Geometry: see drawing. Coordinates: mm, zero at the bounding-box minimum. A direction names the side the tool comes from. Give positions to 0.01 mm unless a question says otherwise; leave off trailing zeros. Order: outer loops, then holes, each group sorted by start corner. A loop starts at its lowest first (then second) coordinate and runs counter-clockwise, first axis right, second up. Notation, with made-up numbers: (88.5, 46) - (120.5, 46) arc R20 cw to (120.5, 66) - close; hole circle Ø2 at (23, 38.5). An arc over 180 degrees is marked (long way). One line per item, written item: value.
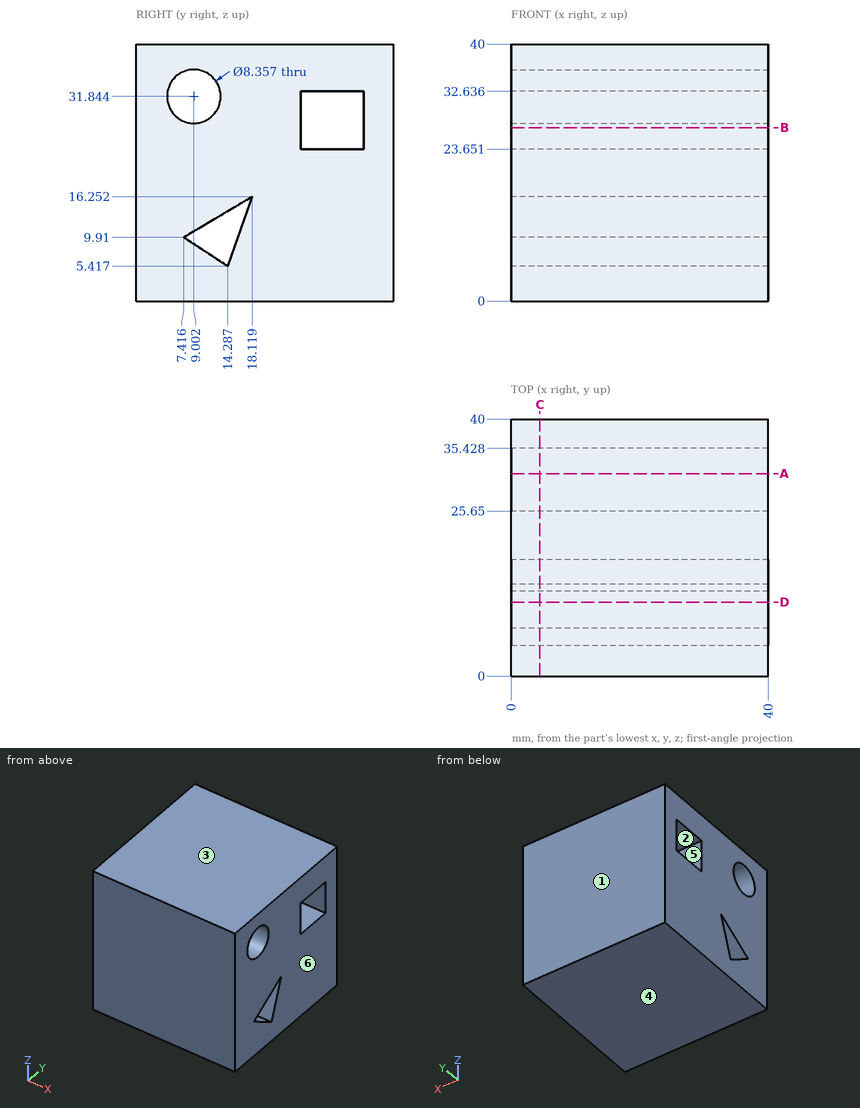
1) Section C-C, the plane x = 4.5. Return loops of the section in (y, z).
Answers below:
outline: (0, 0) - (40, 0) - (40, 40) - (0, 40) - close; hole circle Ø8.36 at (9, 31.84); hole (7.42, 9.91) - (14.29, 5.42) - (18.12, 16.25) - close; hole (25.65, 23.65) - (35.43, 23.65) - (35.43, 32.64) - (25.65, 32.64) - close
2) Section A-A, the plane y = 31.5. Return loops of the section in (x, z).
Answers below:
outline: (0, 0) - (40, 0) - (40, 23.65) - (0, 23.65) - close; (0, 32.64) - (40, 32.64) - (40, 40) - (0, 40) - close
3) Set-up query: the marked faces 5 and 6. Return all of +Z, -Z, +X, -X, +Y, -Y with unobstructed straight access to the full face (end or side cutting, diameter ignored); none if empty.
Answers below:
face 5: +X, -X
face 6: +Z, -Z, +X, +Y, -Y
4) Section B-B, the plane z = 27. Return loops of the section in (x, y), then the cut area to 3 significant figures.
Answers below:
outline: (0, 0) - (40, 0) - (40, 25.65) - (0, 25.65) - close; (0, 35.43) - (40, 35.43) - (40, 40) - (0, 40) - close
area: 1,210 mm^2
5) First-contact query: pin 1 (8 mm diameter, centred on x = 16, z = 16, fed in from -Y). Flat tip, straight axial feed; report the tip coordinate or a pass-through.
Answers below:
pin 1: y = 0
6) Section D-D, the plane y = 11.5. Return loops of the section in (x, z) (1 decimal), then the cut area to 3 significant figures.
Answers below:
outline: (0, 0) - (40, 0) - (40, 7.2) - (0, 7.2) - close; (0, 12.3) - (40, 12.3) - (40, 28.5) - (0, 28.5) - close; (0, 35.2) - (40, 35.2) - (40, 40) - (0, 40) - close
area: 1,130 mm^2
7) Mould query, pull axis Z, two halves, no side actions, for the marked faces 1, 2, 3 and 4. Classes: released by +Z, released by -Z, zero draft, split by the parting line, or undercut.
Answers below:
face 1: zero draft
face 2: undercut
face 3: released by +Z
face 4: released by -Z
8) Material intervals for line 1 along Z through (x, y) = (27, 27); line 2 along Y through (x, z) = (37, 24); line 3 along Z through (x, y) = (7.5, 12) (1 decimal), sorted ascending.
Answers below:
line 1: 0 to 23.65, 32.64 to 40
line 2: 0 to 25.65, 35.43 to 40
line 3: 0 to 6.9, 12.6 to 28.9, 34.8 to 40
